Autodesk Inventor part; units mm, degrees
ref_plane "YZ Plane" through (0, 0, 0) normal (1, 0, 0) x (0, 1, 0)
ref_plane "XZ Plane" through (0, 0, 0) normal (0, 1, 0) x (-1, 0, 0)
ref_plane "XY Plane" through (0, 0, 0) normal (0, 0, 1) x (1, 0, 0)
sketch "Sketch4" plane through (0, 0, 0) normal (0, 1, 0) x (-1, 0, 0)
  line L0 (0, 0) -> (20, 0)
  line L1 (20, 0) -> (20, 80)
  line L2 (20, 80) -> (0, 80)
  line L3 (0, 80) -> (0, 0)
  circle A0 centre (10, 10) radius 2.5
  circle A1 centre (10, 70) radius 2.5
  circle A2 centre (10, 70) radius 2.5
  line L4 (0, 0) -> (20, 0)
  line L5 (20, 0) -> (20, -40)
  line L6 (20, -40) -> (0, -40)
  line L7 (0, -40) -> (0, 0)
  circle A3 centre (10, -30) radius 2.5
  dimension "d0" = 80
  dimension "d3" = 20
  dimension "d4" = 5
  dimension "d5" = 10
  dimension "d6" = 10
  dimension "d7" = 5
  dimension "d8" = 10
  dimension "d9" = 10
  dimension "d12" = 5
  dimension "d13" = 60
  dimension "d16" = 40
  dimension "d17" = 5
  dimension "d18" = 10
  dimension "d19" = 10
extrude "Extrusion3" add sketch "Sketch4" along normal blind 5 contours L3 L2 L1 L0
sketch "Sketch5" plane through (0, 5, 0) normal (0, 1, 0) x (1, 0, 0)
  line L0 (60, -20) -> (-20, -20)
  line L1 (-20, -20) -> (-20, 0)
  line L2 (60, -20) -> (-20, -20)
  line L3 (60, 0) -> (60, -20)
  line L4 (-20, 0) -> (60, 0)
  circle A0 centre (-10, -70) radius 2.5
  circle A1 centre (-10, -10) radius 2.5
  line L5 (0, 0) -> (-20, 0)
  line L6 (-20, 0) -> (-20, -80)
  line L7 (-20, -80) -> (0, -80)
  line L8 (0, -80) -> (0, 0)
  line L9 (-20, 0) -> (0, 0)
  line L10 (0, 0) -> (0, 40)
  line L11 (0, 40) -> (-20, 40)
  line L12 (-20, 40) -> (-20, 0)
  circle A2 centre (-10, 30) radius 2.5
  circle A3 centre (50, -10) radius 2.5
  circle A4 centre (-10, -10) radius 2.5
  circle A5 centre (35, -10) radius 2.5
  dimension "d20" = 40
  dimension "d21" = 5
  dimension "d22" = 10
  dimension "d23" = 10
extrude "Extrusion4" add sketch "Sketch5" against normal blind 5 contours L4 L12 L11 L10
sketch "Sketch6" plane through (0, 5, 0) normal (0, 1, 0) x (1, 0, 0)
  line L0 (-20, 15) -> (-15, 15)
  line L1 (-15, 15) -> (-15, 20)
  line L2 (-15, 20) -> (-20, 20)
  line L3 (-20, 20) -> (-20, 15)
  line L4 (-20, 15) -> (-15, 20) construction
  line L5 (-15, 15) -> (-20, 20) construction
  line L6 (0, 40) -> (-20, 40)
  line L7 (-20, 40) -> (-20, -80)
  line L8 (-20, -25) -> (-15, -25)
  line L9 (-15, -25) -> (-15, -30)
  line L10 (-15, -30) -> (-20, -30)
  line L11 (-20, -30) -> (-20, -25)
  line L12 (-20, -25) -> (-15, -30) construction
  line L13 (-15, -25) -> (-20, -30) construction
  point P0 (0, 0)
  point P1 (-17.5, 17.5)
  point P2 (-17.5, -27.5)
  dimension "d26" = 5
  dimension "d27" = 5
  dimension "d28" = 20
  dimension "d29" = 5
  dimension "d30" = 5
  dimension "d31" = 40
extrude "Extrusion5" cut sketch "Sketch6" against normal through all
sketch "Sketch7" plane through (0, 5, 0) normal (0, 1, 0) x (1, 0, 0)
  circle A0 centre (-10, -52.5) radius 1
  line L0 (-20, -30) -> (-20, -80)
  line L1 (0, 40) -> (-20, 40)
  point P0 (0, 0)
  dimension "d34" = 2
  dimension "d35" = 10
  dimension "d36" = 92.5
extrude "Extrusion6" cut sketch "Sketch7" against normal through all
sketch "Sketch8" plane through (0, 0, 0) normal (0, -1, 0) x (1, 0, 0)
  circle A0 centre (-17.5, -35) radius 1
  line L0 (-20, -20) -> (-20, -40)
  line L1 (-20, -40) -> (0, -40)
  point P0 (0, 0)
  dimension "d39" = 2
  dimension "d40" = 2.5
  dimension "d41" = 5
extrude "Extrusion7" cut sketch "Sketch8" against normal through all
sketch "Sketch9" plane through (0, 0, 0) normal (0, -1, 0) x (1, 0, 0)
  circle A0 centre (-17.5, 38) radius 1
  line L0 (-20, 80) -> (-20, 30)
  line L1 (-20, 30) -> (-15, 30)
  point P0 (0, 0)
  dimension "d44" = 2
  dimension "d45" = 2.5
  dimension "d46" = 8
extrude "Extrusion8" cut sketch "Sketch9" against normal through all
sketch "Sketch10" plane through (0, 5, 0) normal (0, 1, 0) x (1, 0, 0)
  circle A0 centre (50, -70) radius 2.5
  circle A1 centre (-10, -70) radius 2.5
  circle A2 centre (35, -70) radius 2.5
  line L0 (-20, -80) -> (-20, -60)
  line L1 (60, -80) -> (-20, -80)
  line L2 (60, -60) -> (60, -80)
  line L3 (-20, -60) -> (60, -60)
  circle A3 centre (50, -10) radius 2.5
  circle A4 centre (35, -10) radius 2.5
  circle A5 centre (50, -70) radius 2.5
  circle A6 centre (35, -70) radius 2.5
  line L4 (57, 0) -> (27, 0)
  line L5 (27, 0) -> (27, -80)
  line L6 (27, -80) -> (57, -80)
  line L7 (57, -80) -> (57, 0)
  circle A7 centre (50, -10) radius 2.5
  circle A8 centre (-10, -10) radius 2.5
  circle A9 centre (35, -10) radius 2.5
  line L8 (-20, -20) -> (-20, 0)
  line L9 (60, -20) -> (-20, -20)
  line L10 (60, 0) -> (60, -20)
  line L11 (-20, 0) -> (60, 0)
  line L12 (-20, -80) -> (57, -80)
  line L13 (57, -80) -> (57, -60)
  line L14 (57, -60) -> (-20, -60)
  line L15 (-20, -60) -> (-20, -80)
  line L16 (57, 0) -> (27, 0)
  line L17 (27, 0) -> (27, -80)
  line L18 (27, -80) -> (57, -80)
  line L19 (57, -80) -> (57, 0)
  line L20 (-20, 0) -> (57, 0)
  line L21 (57, 0) -> (57, -20)
  line L22 (57, -20) -> (-20, -20)
  line L23 (-20, -20) -> (-20, 0)
  point P0 (0, 0)
extrude "Extrusion9" [suppressed]
sketch "Sketch11" plane through (0, 0, 0) normal (0, -1, 0) x (1, 0, 0)
  line L0 (-20, 55) -> (-15, 55)
  line L1 (-15, 55) -> (-15, 50)
  line L2 (-15, 50) -> (-20, 50)
  line L3 (-20, 50) -> (-20, 55)
  line L4 (-20, 80) -> (0, 80)
  line L5 (-20, 80) -> (-20, 30)
  point P0 (0, 0)
  point P1 (57, 80)
  dimension "d51" = 5
  dimension "d52" = 5
  dimension "d53" = 25
extrude "Extrusion10" cut sketch "Sketch11" against normal through all
sketch "Sketch12" plane through (0, 0, 0) normal (0, -1, 0) x (1, 0, 0)
  line L0 (27, 50) -> (32, 50)
  line L1 (32, 50) -> (32, 55)
  line L2 (32, 55) -> (27, 55)
  line L3 (27, 55) -> (27, 50)
  line L4 (-20, 80) -> (-20, 55)
  line L5 (-20, 80) -> (0, 80)
  point P0 (0, 0)
  point P1 (57, 80)
  dimension "d56" = 5
  dimension "d57" = 5
  dimension "d58" = 47
  dimension "d59" = 25
sketch "Sketch15" plane through (0, 5, 0) normal (0, 1, 0) x (1, 0, 0)
  line L0 (-12.5, -55) -> (-12.5, -103)
  line L1 (-5.379, -59) -> (-8.621, -59)
  circle A0 centre (-10, -10) radius 2.5
  circle A1 centre (-10, -70) radius 2.5
  circle A2 centre (-10, 30) radius 2.5
  line L2 (-20, -50) -> (-15, -50)
  line L3 (-15, -50) -> (-15, -55)
  line L4 (-15, -55) -> (-20, -55)
  line L5 (-20, -55) -> (-20, -80)
  line L6 (-20, -80) -> (0, -80)
  line L7 (0, -80) -> (0, 40)
  line L8 (0, 40) -> (-20, 40)
  line L9 (-20, 20) -> (-15, 20)
  line L10 (-15, 20) -> (-15, 15)
  line L11 (-15, 15) -> (-20, 15)
  line L12 (-20, 15) -> (-20, -25)
  line L13 (-20, -25) -> (-15, -25)
  line L14 (-15, -25) -> (-15, -30)
  line L15 (-15, -30) -> (-20, -30)
  line L16 (-20, -30) -> (-20, -50)
  circle A3 centre (-10, -52.5) radius 1
  circle A4 centre (-17.5, 35) radius 1
  circle A5 centre (-17.5, -38) radius 1
  line L17 (-20, -80) -> (60, -80)
  line L18 (60, -80) -> (60, -60)
  line L19 (60, -60) -> (-20, -60)
  line L20 (-20, -60) -> (-20, -80)
  line L21 (60, -80) -> (40, -80)
  line L22 (40, -80) -> (40, 0)
  line L23 (40, 0) -> (60, 0)
  line L24 (60, 0) -> (60, -80)
  line L25 (-20, 0) -> (60, 0)
  line L26 (60, 0) -> (60, -20)
  line L27 (60, -20) -> (-20, -20)
  line L28 (-20, -20) -> (-20, 0)
  circle A6 centre (37, -70) radius 2.5
  circle A7 centre (52, -70) radius 2.5
  circle A8 centre (52, -10) radius 2.5
  circle A9 centre (37, -10) radius 2.5
  line L29 (-20, 40) -> (-20, 20)
  point P0 (0, 0)
  dimension "d69" = 20
  dimension "d70" = 80
  dimension "d71" = 20
  dimension "d72" = 80
  dimension "d73" = 5
  dimension "d74" = 5
  dimension "d75" = 8
  dimension "d76" = 23
  dimension "d77" = 5
  dimension "d78" = 5
  dimension "d79" = 8
  dimension "d80" = 23
  dimension "d81" = 10
  dimension "d82" = 10
  dimension "d90" = 20
extrude "Extrusion14" add sketch "Sketch15" against normal blind 5 contours L19 L7 L6 L0 | L0 L6 L5 L19 | L19 L22 L17 L7 | L27 L12 L25 L7 | L7 L25 L22 L27 | L22 L27 L24 L19 | L19 L18 L17 L22 | L22 L23 L24 L27
sketch "Sketch16" plane through (0, 5, 0) normal (0, 1, 0) x (1, 0, 0)
  line L0 (45, -55) -> (40, -55)
  line L1 (40, -55) -> (40, -50)
  line L2 (40, -50) -> (45, -50)
  line L3 (45, -50) -> (45, -55)
  line L4 (40, -20) -> (40, -60)
  line L5 (-20, -80) -> (60, -80)
  point P0 (0, 0)
  dimension "d85" = 5
  dimension "d86" = 5
  dimension "d87" = 25
extrude "Extrusion15" cut sketch "Sketch16" against normal through all
equation "\"d37\" = d36"
properties part number "holdersupport" material "Wood (Birch)"
For this review, take the finished solid that the model builds, in its own axes (mm). A direction names the side the tool comes from. Coordinates: 2 decimals unless noted, no trailing zeros. Order: outer loops, then holes, each group sorted by start corner. A loop starts at its lowest first (then second) coordinate and runs counter-clockwise, first axis right, second up. Notation, with made-up numbers: (57.5, 53.25) - (71.5, 53.25) arc R24 ccw to (71.5, 89.25) - close; hole circle Ø10 at (21, 88). An arc over 180 degrees is marked (long way). Answer as CSV lines item,"result". Start each with the question number.
1) Add section D-D (x = 52). State the section outline as (y, z) points, then the cut area to 3 significant figures.
2) Machinability: for faces 4 (the flat face through (40, 3, 58)), 5 (the flat face through (-18, 3, -15)), 6 (the flat face through (0, 2, -20)), which of the approach directions +Z, -Z, +X, -X, +Y, -Y give a long, thin tool a straight path to every point of the face, cutting with its end or side? Answer none if there is none.
3) Add section A-A (z = 23.5). State the section outline as (x, y) points, then the cut area to 3 significant figures.
4) Add section B-B (x = 8). State the section outline as (y, z) points, then the cut area to 3 significant figures.
5) To check wall thickness, follow line 1 along Z through (x, y) = (-10, 1.7); line 2 along X through (y, z) = (4.65, 31); line 3 along Z through (x, y) = (5.5, 4.6). State the ranges of each line that lie inside material, in increasing order. Write a range as [from, to].
6) Insertion check: P1, Ø3, axis at y = 4, z = -5, coming from the +X side; P2, Ø2.5, axis at y = 1.5, z = -18.5, coming from the -X side; P3, Ø2.5, axis at x = 25, y = 3, coming from the -Z side. Each pin has a flat end and moves straight along its axis. Give the tip position at first contact, or say it passes through.
7) Draft analysis for pull direction Z (two halves, no side actions). For faces 1 (the flat face through (-15, 3, -17)), 2 (the flat face through (-10, 3, -40)), 3 (the flat face through (-6, 5, 34)), state which applies: +Z half, -Z half, draft (parallel to the pull), parting line (faces both ways), or undercut.
8) Add section C-C (z = 10). State the section outline as (x, y) points, then the cut area to 3 significant figures.
Result:
1,outline,"(0, 0) - (5, 0) - (5, 7.5) - (0, 7.5) - close; (0, 12.5) - (5, 12.5) - (5, 67.5) - (0, 67.5) - close; (0, 72.5) - (5, 72.5) - (5, 80) - (0, 80) - close"
1,area,"350 mm^2"
2,face 4,"+Y, -Y"
2,face 5,"-X, +Y, -Y"
2,face 6,"-Z, +X, +Y, -Y"
3,outline,"(-20, 0) - (0, 0) - (0, 5) - (-20, 5) - close; (40, 0) - (60, 0) - (60, 5) - (40, 5) - close"
3,area,"200 mm^2"
4,outline,"(0, 0) - (5, 0) - (5, 20) - (0, 20) - close; (0, 60) - (5, 60) - (5, 80) - (0, 80) - close"
4,area,"200 mm^2"
5,line 1,"[-40, -32.5], [-27.5, 7.5], [12.5, 51.5], [53.5, 67.5], [72.5, 80]"
5,line 2,"[-20, 0], [40, 60]"
5,line 3,"[0, 20], [60, 80]"
6,P1,"x = 0"
6,P2,"x = -15"
6,P3,"z = 0"
7,face 1,"undercut"
7,face 2,"-Z half"
7,face 3,"draft"
8,outline,"(-20, 0) - (-12.5, 0) - (-12.5, 5) - (-20, 5) - close; (-7.5, 0) - (34.5, 0) - (34.5, 5) - (-7.5, 5) - close; (39.5, 0) - (49.5, 0) - (49.5, 5) - (39.5, 5) - close; (54.5, 0) - (60, 0) - (60, 5) - (54.5, 5) - close"
8,area,"325 mm^2"
